Design review of the part built by this model. Coordinates are the model's own, in mm. Face numbers are marked on the shaded views. A direction names the side the tool comes from. Coordinates: 2 decimals unless noted, no trailing zeros. Loops run counter-clockwise (first coordinate to the right, second up) from the corner with the lowest first, then second, coordinate; pieces in that order, holes last. Notation, with made-up numbers: (79, 22.5) -> (99, 22.5) arc R17 cw to (99, 33.5) -> close; hole circle Ø10 at (78.25, 87). An arc over 180 degrees is marked (long way). Use CSV: the item, a comma, the result in double quotes.
```python
from build123d import *

# Parameters (mm, degrees)
F0_W     = 4
F0_H     = 3
F1_DEPTH = 36
F2_R     = 15
F3_DEPTH = 25
F4_R     = 1.49999
F5_R     = 0.5
F6_SIZE  = 0.4


# Not quite as in the source:
# - a fillet or chamfer is up to 0.001 mm smaller than in the source, because OpenCascade refuses the exact size
# - a feature names something its author has since deleted; it is built from what else it names


with BuildPart() as f1:
    # F0 (on Top) → F1 (new body)
    with BuildSketch(Plane.XY):
        Polygon((-3, 0), (0, 0), (0, 3), (0, 18.6), (25.8, 18.6), (25.8, -21.4), (64.8, -21.4), (64.8, -18.4), (28.8, -18.4), (28.8, 21.6), (-3, 21.6), align=None)
        with Locations((2, 1.5)):
            Rectangle(F0_W, F0_H)
    extrude(amount=F1_DEPTH)

    # F2 (on face) → F3 (cut)
    with BuildSketch(Plane(origin=(0, -18.4, 0), x_dir=(-1, 0, 0), z_dir=(0, 1, 0))):
        with Locations((-46.8, 18)):
            Circle(F2_R)
    extrude(amount=-F3_DEPTH, mode=Mode.SUBTRACT)

    # F4 (radius 1.5 in the source; OpenCascade refuses exactly that, so slightly less here)
    f4_edges = [f1.edges().sort_by_distance(p)[0] for p in [
        (-3, 0, 18),
        (-3, 21.6, 18),
        (28.8, 21.6, 18),
        (28.8, -18.4, 18),
        (25.8, -21.4, 18),
        (4, 3, 18),
        (4, 0, 18),
        (64.8, -21.4, 18),
        (64.8, -18.4, 18),
    ]]
    fillet(f4_edges, radius=F4_R)

    # F5
    f5_edges = [f1.edges().sort_by_distance(p)[0] for p in [
        (0, 18.6, 18),
        (25.8, 18.6, 18),
        (0, 3, 18),
    ]]
    fillet(f5_edges, radius=F5_R)

    # F6
    f6_edges = [f1.edges().sort_by_distance(p)[0] for p in [
        (1.500005, 3, 36),
        (0.146447, 3.146447, 36),
        (3.560663, 2.560663, 36),
        (0, 10.8, 36),
        (4, 1.5, 36),
        (0.146447, 18.453553, 36),
        (3.560663, 0.439337, 36),
        (12.9, 18.6, 36),
        (0.5, 0, 36),
        (25.653553, 18.453553, 36),
        (-2.560663, 0.439337, 36),
        (25.8, -0.900005, 36),
        (-3, 10.8, 36),
        (26.239337, -20.960663, 36),
        (-2.560663, 21.160663, 36),
        (45.3, -21.4, 36),
        (12.9, 21.6, 36),
        (64.360663, -20.960663, 36),
        (28.360663, 21.160663, 36),
        (64.8, -19.9, 36),
        (28.8, 1.6, 36),
        (64.360663, -18.839337, 36),
        (29.239337, -17.960663, 36),
        (46.8, -18.4, 36),
        (1.500005, 3, 0),
        (0.146447, 3.146447, 0),
        (3.560663, 2.560663, 0),
        (0, 10.8, 0),
        (4, 1.5, 0),
        (0.146447, 18.453553, 0),
        (3.560663, 0.439337, 0),
        (12.9, 18.6, 0),
        (0.5, 0, 0),
        (25.653553, 18.453553, 0),
        (-2.560663, 0.439337, 0),
        (25.8, -0.900005, 0),
        (-3, 10.8, 0),
        (26.239337, -20.960663, 0),
        (-2.560663, 21.160663, 0),
        (45.3, -21.4, 0),
        (12.9, 21.6, 0),
        (64.360663, -20.960663, 0),
        (28.360663, 21.160663, 0),
        (64.8, -19.9, 0),
        (28.8, 1.6, 0),
        (64.360663, -18.839337, 0),
        (29.239337, -17.960663, 0),
        (46.8, -18.4, 0),
        (61.8, -18.4, 18),
        (61.8, -21.4, 18),
    ]]
    chamfer(f6_edges, length=F6_SIZE)


solid = f1.part
```
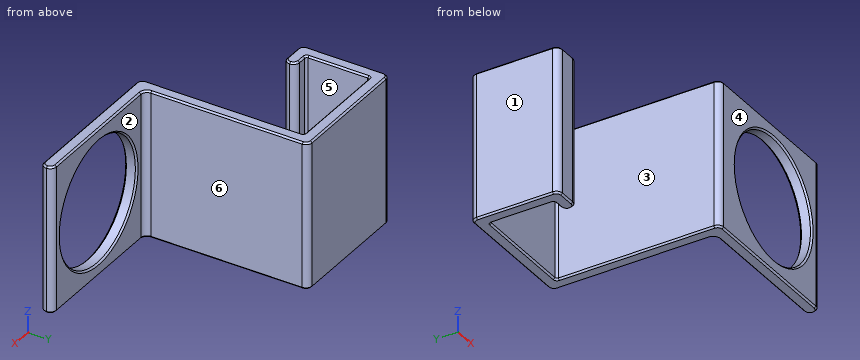
Item 1: Machinability: for the marked faces 1, 2 and 3, which of the approach directions +Z, -Z, +X, -X, +Y, -Y give a long, thin tool a straight path to every point of the face, cutting with its end or side? Answer none if there is none.
Checked values:
face 1,"+Z, -Z, -X, +Y, -Y"
face 2,"+Z, -Z, +X, +Y"
face 3,"+Z, -Z, -Y"
Item 2: Add section C-C (x = 46.8). Give the boundary of the cut face in (y, z), then the cut area to 3 significant figures.
Checked values:
outline,"(-21.4, 0.4) -> (-21, 0) -> (-18.8, 0) -> (-18.4, 0.4) -> (-18.4, 2.6) -> (-18.8, 3) -> (-21, 3) -> (-21.4, 2.6) -> close; (-21.4, 33.4) -> (-21, 33) -> (-18.8, 33) -> (-18.4, 33.4) -> (-18.4, 35.6) -> (-18.8, 36) -> (-21, 36) -> (-21.4, 35.6) -> close"
area,"17.4 mm^2"
Item 3: Add section A-A (y = 15). Give the boundary of the cut face in (x, z).
Checked values:
outline,"(-3, 0.4) -> (-2.6, 0) -> (-0.4, 0) -> (0, 0.4) -> (0, 35.6) -> (-0.4, 36) -> (-2.6, 36) -> (-3, 35.6) -> close; (25.8, 0.4) -> (26.2, 0) -> (28.4, 0) -> (28.8, 0.4) -> (28.8, 35.6) -> (28.4, 36) -> (26.2, 36) -> (25.8, 35.6) -> close"
Item 4: Add section D-D (x = 24). Give the boundary of the cut face in (y, z), then the cut area to 3 significant figures.
Checked values:
outline,"(18.6, 0.4) -> (19, 0) -> (21.2, 0) -> (21.6, 0.4) -> (21.6, 35.6) -> (21.2, 36) -> (19, 36) -> (18.6, 35.6) -> close"
area,"108 mm^2"
Item 5: To check wall thickness, follow line 1 along X through (y, z) = (12, 4); line 2 along Z through (x, y) = (46.8, -20.1); line 3 along Y through (x, z) = (20.5, 32.5). State the ranges of each line that lie inside material, in increasing order.
Checked values:
line 1,"-3 to 0, 25.8 to 28.8"
line 2,"0 to 3, 33 to 36"
line 3,"18.6 to 21.6"
Item 6: Clearance check with flat-ended pins moving along their axes: pin 1 (12 mm diameter, centred on x = 47.5, z = 7, fed in from -Y); pin 2 (6 mm diameter, centred on x = 11, z = 18, fed in from -Y); pin 3 (7.5 mm diameter, centred on y = 9.5, z = 19, fed in from +X); pin 4 (16.5 mm diameter, centred on x = 45, z = 10, fed in from +Y). State where each tip first meets the part, or that it passes through.
Checked values:
pin 1,"y = -21.4"
pin 2,"y = 18.6"
pin 3,"x = 28.8"
pin 4,"y = -18.4"
Item 7: Draft analysis for pull direction X (two halves, no side actions). For the marked faces 4, 5 and 6, state which applies: pulls with the +X half, pulls with the -X half, needs draft (parallel to the pull), parting line crosses it, or undercut.
Checked values:
face 4,"needs draft"
face 5,"undercut"
face 6,"pulls with the +X half"
